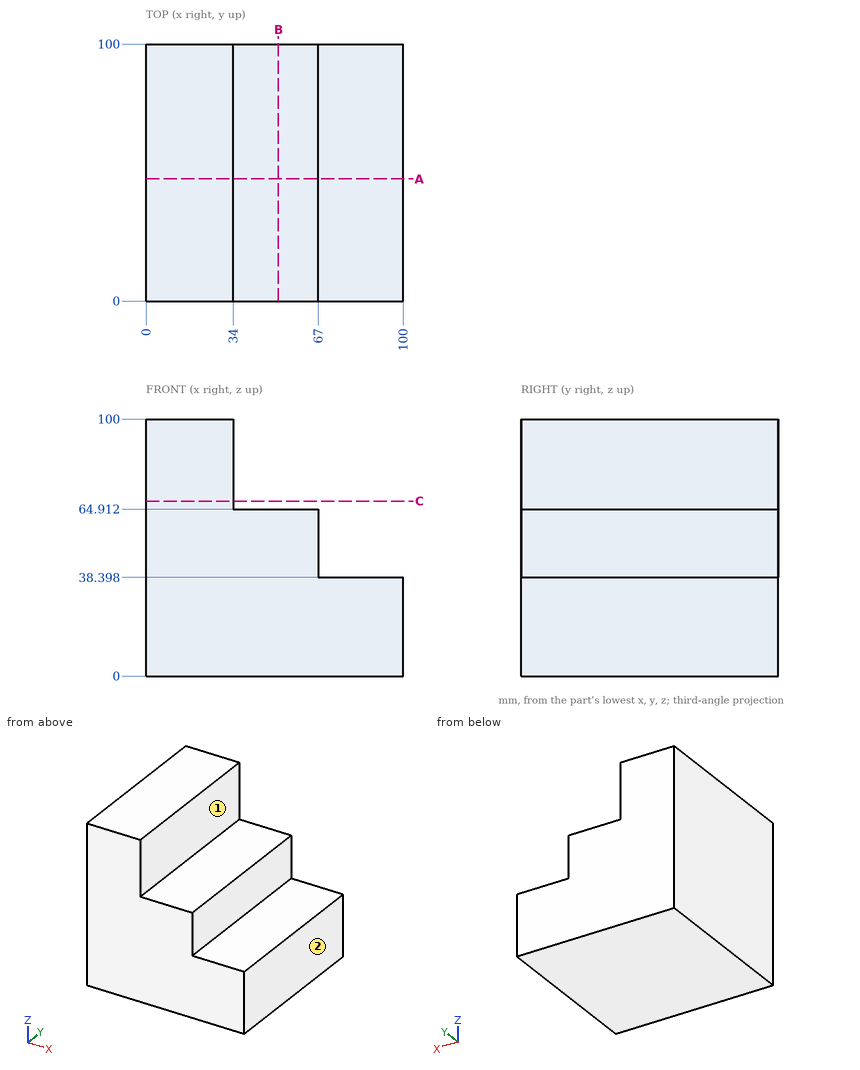
Here's the drawing with two shaded views (mm, measured from the low corner). I have some questions. A direction names the side the tool comes from. Coordinates: 2 decimals unless noted, no trailing zeros. Write each loop counter-clockwise with the first axis right and the second up, starting at its lowest first coordinate (ties: lowest second). Pieces come first, ordered by that corner, then holes. Notation, with made-up numbers: (62.25, 11.25) -> (88.25, 11.25) arc R30 ccw to (88.25, 42.25) -> close; hole circle Ø8 at (-15.5, 64.5). An arc over 180 degrees is marked (long way). Write item = value, one per line. Start each with the question number.
(1) Which directions (+Z, -Z, +X, -X, +Y, -Y) give clear straight access to the entire face, cutting with the end or side of a thin tool? Please do the marked faces 1 and 2.
(2) I need wall thicknesses on line 1 (Z direction, x = 73.5, y = 47); line 2 (Z direction, x = 54.5, y = 21); line 3 (X direction, y = 19, z = 71). Which ranges of each line are inside material? Lowest first, please. Write a range as [from, to].
(3) I want a section at B-B (x = 51.5). Please give me the cut outline in (y, z), plus the area to 3 significant figures.
(4) Will these pins go through, and if not, where does the flat tip stop? pin 1 (16.5 mm diameter, centred on x = 80.5, y = 49, fed in from +Z); pin 2 (10 mm diameter, centred on x = 46.5, y = 31.5, fed in from +Z); pin 3 (1 mm diameter, centred on y = 74, z = 80, fed in from +X).
(5) I want a section at C-C (z = 68). Please give me the cut outline in (x, y), plus the area to 3 significant figures.
(6) I want a section at A-A (y = 47.5). Please give me the cut outline in (x, z), plus the area to 3 significant figures.
Result set:
q1.face_1 = +Z, +X, +Y, -Y
q1.face_2 = +Z, -Z, +X, +Y, -Y
q2.line_1 = [0, 38.4]
q2.line_2 = [0, 64.91]
q2.line_3 = [0, 34]
q3.outline = (0, 0) -> (100, 0) -> (100, 64.91) -> (0, 64.91) -> close
q3.area = 6,490 mm2
q4.pin_1 = 38.4
q4.pin_2 = 64.91
q4.pin_3 = 34
q5.outline = (0, 0) -> (34, 0) -> (34, 100) -> (0, 100) -> close
q5.area = 3,400 mm2
q6.outline = (0, 0) -> (100, 0) -> (100, 38.4) -> (67, 38.4) -> (67, 64.91) -> (34, 64.91) -> (34, 100) -> (0, 100) -> close
q6.area = 6,810 mm2
